Geometry check sheet. Reference: the model listing, model coordinates, mm. A direction names the side the tool comes from. Round coordinates to 2 decimals unless told otherwise and drop trailing zeros. Loops run counter-clockwise (first coordinate to the right, second up) from the corner with the lowest first, then second, coordinate; pieces in that order, holes last. Notation, with made-up numbers: (5, 75.25) -> (28, 75.25) arc R18 cw to (28, 105.25) -> close; hole circle Ø3 at (4, -22). An arc over 180 degrees is marked (long way). Use a Markdown table: item, result. Add a question column.
Q1. Material ranges on L1, parallel to Y at x = 3, z = -0.85; L2, parallel to Z at x = 19, y = 34; L3, parallel to Y at x = 3, z = 0.7, recorded low to high.
Q2. Sectioned sample at C-C, the plane y = 16.5. Enter the section's corners in (x, z).
Q3. Set-up check for faces 1 (the face through (1, 2, -4)), 2 (the face through (0.615, 0.751, -2.028)), 3 (the face through (6, 13, 1)): record each of +Z, -Z, +X, -X, +Y, -Y from which the full face is reachable in a straight line by a thin tool's end or side.
Q4. Sectioned sample at D-D, the plane x = 10.5. Enter the section's corners in (y, z), then the cut area to 3 significant figures.
Q5. Gauge pin test, flat ends, axial feed: P1, Ø10, axis at x = 23.5, y = 24, coming from the -Z side; P2, Ø0.6, axis at y = 16.5, z = 1, coming from the +X side; P3, Ø2.5, axis at x = 3, y = 0, coming from the +Z side; P4, Ø4.5, axis at x = 3, y = 0, coming from the -Z side. Record the tip position at first contact, or that the pin passes through.
Q6. Sectioned sample at A-A, the plane z = 0.6. Enter the section's corners in (x, y), then the cut area to 3 significant figures.
Q7. Sectioned sample at B-B, the plane x = 3. Enter the section's corners in (y, z).
Q8. Release check for a two-part mould opening along Y. For faces 4 (the face through (32.677, 45.845, 0.986)), 5 (the face through (32.55, 33.16, 0.99)), 6 (the face through (2, -1, 0)) record: released by +Y, released by -Y, zero draft, split by the parting line, or undercut.
```python
from build123d import *

# Parameters (mm, degrees)
BOSS_EXTRUDE1_DEPTH = 2
BOSS_EXTRUDE2_START = -6
SKETCH2_R           = 3
BOSS_EXTRUDE2_DEPTH = 6
SKETCH3_R           = 2.5
CUT_EXTRUDE1_DEPTH  = 4
SKETCH4_R           = 1
CUT_EXTRUDE2_DEPTH  = 2


with BuildPart() as part:
    # Sketch1 → Boss-Extrude1 (new body)
    with BuildSketch(Plane.XY):
        with BuildLine():
            Line((0, 42.082464074), (0, 0))
            ThreePointArc((0, 0), (3, -3), (6, 0))
            Line((6, 0), (6, 26.214927972))
            Line((6, 26.214927972), (26.736481777, 29.871329194))
            ThreePointArc((26.736481777, 29.871329194), (32.614961131, 33.237711964), (34.999006977, 39.578483044))
            ThreePointArc((34.999006977, 39.578483044), (32.614961131, 45.919254124), (26.736481777, 49.285636894))
            Line((26.736481777, 49.285636894), (11.736481777, 51.930541604))
            ThreePointArc((11.736481777, 51.930541604), (3.572123903, 49.742908505), (0, 42.082464074))
        make_face()
    extrude(amount=BOSS_EXTRUDE1_DEPTH)

    # Sketch2 → Boss-Extrude2 (add)
    with BuildSketch(Plane.XY.offset(2).offset(BOSS_EXTRUDE2_START)):
        with Locations((3, 0)):
            Circle(SKETCH2_R)
    extrude(amount=BOSS_EXTRUDE2_DEPTH)

    # Sketch3 → Cut-Extrude1 (cut)
    with BuildSketch(Plane(origin=(0, 0, -4), x_dir=(-1, 0, 0), z_dir=(0, 0, -1))):
        with Locations((-3, 0)):
            Circle(SKETCH3_R)
    extrude(amount=-CUT_EXTRUDE1_DEPTH, mode=Mode.SUBTRACT)

    # Sketch4 → Cut-Extrude2 (cut)
    with BuildSketch(Plane(origin=(0, 0, 0), x_dir=(-1, 0, 0), z_dir=(0, 0, -1))):
        with Locations((-3, 0)):
            Circle(SKETCH4_R)
    extrude(amount=-CUT_EXTRUDE2_DEPTH, mode=Mode.SUBTRACT)


solid = part.part
```
Values:
| question | item | result |
|---|---|---|
| 1 | L1 | -3 to -2.5, 2.5 to 3 |
| 1 | L2 | 0 to 2 |
| 1 | L3 | -3 to -1, 1 to 49.22 |
| 2 | outline | (0, 0) -> (6, 0) -> (6, 2) -> (0, 2) -> close |
| 3 | face 1 | -Z, +X, -X, +Y, -Y |
| 3 | face 2 | -Z |
| 3 | face 3 | +Z, -Z, +X, -Y |
| 4 | outline | (27.01, 0) -> (52.07, 0) -> (52.07, 2) -> (27.01, 2) -> close |
| 4 | area | 50.1 mm^2 |
| 5 | P1 | through |
| 5 | P2 | x = 6 |
| 5 | P3 | z = 2 |
| 5 | P4 | z = 0 |
| 6 | outline | (0, 0) arc R3 ccw to (6, 0) -> (6, 26.21) -> (26.74, 29.87) arc R10 ccw to (35, 39.58) arc R10 ccw to (26.74, 49.29) -> (11.74, 51.93) arc R10 ccw to (0, 42.08) -> close; hole circle Ø2 at (3, 0) |
| 6 | area | 899 mm^2 |
| 7 | outline | (-3, -4) -> (-2.5, -4) -> (-2.5, 0) -> (-1, 0) -> (-1, 2) -> (-3, 2) -> close; (1, 0) -> (2.5, 0) -> (2.5, -4) -> (3, -4) -> (3, 0) -> (49.22, 0) -> (49.22, 2) -> (1, 2) -> close |
| 8 | face 4 | released by +Y |
| 8 | face 5 | released by -Y |
| 8 | face 6 | undercut |
